Geometry: final body of the model. Coordinates: model frame, mm. Give positions to 0.01 mm unless a question says otherwise; leave off trailing zeros. Order: outer loops, then holes, each group sorted by start corner. A loop starts at its lowest first (then second) coordinate and runs counter-clockwise, first axis right, second up. Notation, with made-up numbers: (-6.5, 11) -> (30.5, 11) arc R14 ccw to (30.5, 34) -> close; hole circle Ø3 at (72.5, 51). An arc over 180 degrees is marked (long way). Answer in a Markdown table with one row per item. Add a question column.
Q1. Cut plane C-C on y = -90. Return the cut outline in (x, z).
Q2. Cut plane B-B on x = -142.5. Return the cut outline in (y, z).
Q3. Cut plane A-A on z = 2.35. Return the cut outline in (x, y), and give its area (3 significant figures).
Q4. Contact query for flat-ended pins moving along their axis: P1, Ø2.5, axis at y = -92.5, z = 2.5, coming from the -X side; P2, Ø1.5, axis at y = -115.5, z = 1.5, coming from the -X side; P3, Ø1.5, axis at x = -67.5, z = 3.5, coming from the -Y side. Output: stop coordinate, or through.
Q5. Line query: line 1 along X through (y, z) = (-86, 1.05); line 2 along X through (y, z) = (-74, 3.65); line 3 along Y through (x, z) = (-140, 0.75). Output: solid intervals per line, ascending. Write a range as from..to.
from build123d import *

# Parameters (mm, degrees)
SKIZZE1_W                       = 85
SKIZZE1_H                       = 38
SKIZZE1_W_2                     = 60
SKIZZE1_H_2                     = 5
SKIZZE1_W_3                     = 5
SKIZZE1_H_3                     = 9
AUFSATZ_LINEAR_AUSTRAGEN1_DEPTH = 5


with BuildPart() as part:
    # Skizze1 → Aufsatz-Linear austragen1 (new body)
    with BuildSketch(Plane.XY):
        with Locations((-109.774617185, -94.268113146)):
            Rectangle(SKIZZE1_W, SKIZZE1_H)
        with Locations((-109.835742472, -115.768113146)):
            Rectangle(SKIZZE1_W_2, SKIZZE1_H_2)
        with Locations((-154.774617185, -108.768113146)):
            Rectangle(SKIZZE1_W_3, SKIZZE1_H_3)
        with Locations((-154.774617185, -79.768113146)):
            Rectangle(SKIZZE1_W_3, SKIZZE1_H_3)
        with Locations((-109.835742472, -72.768113146)):
            Rectangle(SKIZZE1_W_2, SKIZZE1_H_2)
        with Locations((-64.774617185, -79.768113146)):
            Rectangle(SKIZZE1_W_3, SKIZZE1_H_3)
        with Locations((-64.774617185, -108.768113146)):
            Rectangle(SKIZZE1_W_3, SKIZZE1_H_3)
    extrude(amount=AUFSATZ_LINEAR_AUSTRAGEN1_DEPTH)


solid = part.part
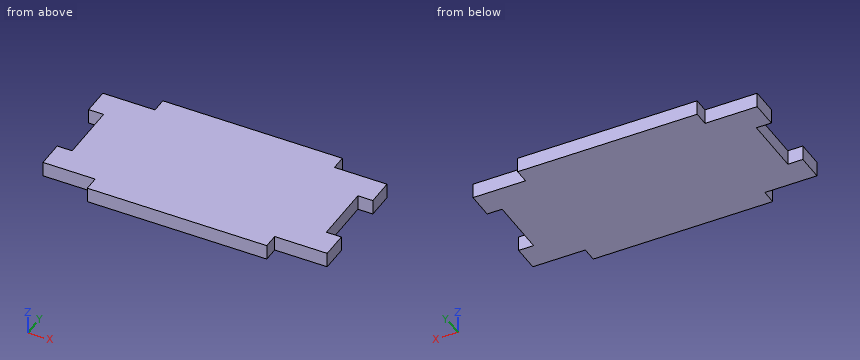
Completed:
| question | item | result |
|---|---|---|
| 1 | outline | (-152.27, 0) -> (-67.27, 0) -> (-67.27, 5) -> (-152.27, 5) -> close |
| 2 | outline | (-113.27, 0) -> (-75.27, 0) -> (-75.27, 5) -> (-113.27, 5) -> close |
| 3 | outline | (-157.27, -113.27) -> (-139.84, -113.27) -> (-139.84, -118.27) -> (-79.84, -118.27) -> (-79.84, -113.27) -> (-62.27, -113.27) -> (-62.27, -104.27) -> (-67.27, -104.27) -> (-67.27, -84.27) -> (-62.27, -84.27) -> (-62.27, -75.27) -> (-79.84, -75.27) -> (-79.84, -70.27) -> (-139.84, -70.27) -> (-139.84, -75.27) -> (-157.27, -75.27) -> (-157.27, -84.27) -> (-152.27, -84.27) -> (-152.27, -104.27) -> (-157.27, -104.27) -> close |
| 3 | area | 4,010 mm² |
| 4 | P1 | stops at x = -152.27 |
| 4 | P2 | stops at x = -139.84 |
| 4 | P3 | stops at y = -113.27 |
| 5 | line 1 | x = -152.27..-67.27 |
| 5 | line 2 | x = -139.84..-79.84 |
| 5 | line 3 | y = -113.27..-75.27 |
